Build history of the part. All positions in model axes, mm. A direction names the side the tool comes from. Coordinates: 2 decimals unless noted, no trailing zeros. Order: outer loops, then holes, each group sorted by start corner. A loop starts at its lowest first (then second) coordinate and runs counter-clockwise, first axis right, second up. Notation, with made-up numbers: M -29.75,-24.5 L -6.75,-24.5 A19 cw -6.75,-19.5 Z; hole C 18.5,32 d11. An arc over 180 degrees is marked long. Use a Markdown table: item, result. Add a question column.
from build123d import *

# Parameters (mm, degrees)
BOSS_EXTRUDE1_DEPTH = 152.4
BOSS_EXTRUDE2_DEPTH = 12.7
SKETCH3_R           = 2.5
CUT_EXTRUDE1_DEPTH  = 25
SKETCH4_R           = 3.5
CUT_EXTRUDE2_DEPTH  = 2


with BuildPart() as part:
    # Sketch1 → Boss-Extrude1 (new body)
    with BuildSketch(Plane(origin=(0, 0, 0), x_dir=(0, 1, 0), z_dir=(0, 0, 1))):
        with BuildLine():
            Line((-94.231538291, 5), (-88.9, 5))
            Line((-88.9, 5), (-88.9, 19.05))
            Line((-88.9, 19.05), (-215.9, 19.05))
            Line((-215.9, 19.05), (-215.9, -7.7))
            ThreePointArc((-215.9, -7.7), (-208.57766953, -25.37766953), (-190.9, -32.7))
            Line((-190.9, -32.7), (-152.8, -32.7))
            Line((-152.8, -32.7), (-152.8, -20))
            Line((-152.8, -20), (-170.3, -20))
            ThreePointArc((-170.3, -20), (-175.603300859, -17.803300859), (-177.8, -12.5))
            Line((-177.8, -12.5), (-177.8, -7.5))
            ThreePointArc((-177.8, -7.5), (-175.603300859, -2.196699141), (-170.3, 0))
            Line((-170.3, 0), (-141.9, 0))
            Line((-141.9, 0), (-144.231538291, 5))
            Line((-144.231538291, 5), (-133.568461709, 5))
            Line((-133.568461709, 5), (-135.9, 0))
            Line((-135.9, 0), (-91.9, 0))
            Line((-91.9, 0), (-94.231538291, 5))
        make_face()
        with BuildLine():
            Line((-35.9, 0), (-7.5, 0))
            ThreePointArc((-7.5, 0), (-2.196699141, -2.196699141), (0, -7.5))
            Line((0, -7.5), (0, -12.5))
            ThreePointArc((0, -12.5), (-2.196699141, -17.803300859), (-7.5, -20))
            Line((-7.5, -20), (-25, -20))
            Line((-25, -20), (-25, -32.7))
            Line((-25, -32.7), (13.1, -32.7))
            ThreePointArc((13.1, -32.7), (30.77766953, -25.37766953), (38.1, -7.7))
            Line((38.1, -7.7), (38.1, 19.05))
            Line((38.1, 19.05), (-88.9, 19.05))
            Line((-88.9, 19.05), (-88.9, 5))
            Line((-88.9, 5), (-83.568461709, 5))
            Line((-83.568461709, 5), (-85.9, 0))
            Line((-85.9, 0), (-41.9, 0))
            Line((-41.9, 0), (-44.231538291, 5))
            Line((-44.231538291, 5), (-33.568461709, 5))
            Line((-33.568461709, 5), (-35.9, 0))
        make_face()
    extrude(amount=BOSS_EXTRUDE1_DEPTH)

    # Sketch2 → Boss-Extrude2 (add)
    with BuildSketch(Plane(origin=(0, 0, 0), x_dir=(1, 0, 0), z_dir=(0, 0, -1))):
        Polygon((-19.05, 215.9), (-19.05, -38.1), (7.7, -38.1), (32.7, 25), (32.7, 152.8), (32.7, 190.9), (7.7, 215.9), align=None)
    extrude(amount=-BOSS_EXTRUDE2_DEPTH)

    # Sketch3 → Cut-Extrude1 (cut)
    with BuildSketch(Plane.YZ):
        with Locations(Location((-107.285735893, 82.55, 0), (0, 0, 270))):
            Circle(SKETCH3_R)
        with Locations(Location((-107.285735893, 127.55, 0), (0, 0, 270))):
            Circle(SKETCH3_R)
        with Locations(Location((-107.285735893, 37.55, 0), (0, 0, 270))):
            Circle(SKETCH3_R)
        with Locations(Location((-70.514264107, 37.55, 0), (0, 0, 180))):
            Circle(SKETCH3_R)
        with Locations(Location((-70.514264107, 82.55, 0), (0, 0, 180))):
            Circle(SKETCH3_R)
        with Locations(Location((-70.514264107, 127.55, 0), (0, 0, 180))):
            Circle(SKETCH3_R)
    extrude(amount=-CUT_EXTRUDE1_DEPTH, mode=Mode.SUBTRACT)

    # Sketch4 → Cut-Extrude2 (cut)
    with BuildSketch(Plane.YZ):
        with Locations(Location((-107.285735893, 127.55, 0), (0, 0, 270))):
            Circle(SKETCH4_R)
        with Locations(Location((-107.285735893, 82.55, 0), (0, 0, 270))):
            Circle(SKETCH4_R)
        with Locations(Location((-107.285735893, 37.55, 0), (0, 0, 270))):
            Circle(SKETCH4_R)
        with Locations(Location((-70.514264107, 37.55, 0), (0, 0, 270))):
            Circle(SKETCH4_R)
        with Locations(Location((-70.514264107, 82.55, 0), (0, 0, 270))):
            Circle(SKETCH4_R)
        with Locations(Location((-70.514264107, 127.55, 0), (0, 0, 270))):
            Circle(SKETCH4_R)
    extrude(amount=-CUT_EXTRUDE2_DEPTH, mode=Mode.SUBTRACT)


solid = part.part
(1) Slice it at C-C on z = 37.55. State how many separate pieces and enclosed holes the cut face has, and give its area (3 significant figures).
(2) Slice it at D-D on x = 22.5. Give the cut face in (y, z), and give its area (3 significant figures).
(3) Mould opens along Z. For faces 1 (the flat face through (-11, -91, 152.4)), 2 (the flat face through (26, -152.8, 82)), 3 (the flat face through (-2, -106, 85)) say: released by +Z, released by -Z, zero draft, split by the parting line, or undercut.
(4) Drop flat-ended pins along their axis: P1, Ø8.5, axis at y = -41, z = 107.5, coming from the +X side; P2, Ø1.5, axis at x = 14.5, z = 39, coming from the +Y side; P3, Ø12, axis at x = 23, z = 98, coming from the -Y side. Give the stop position or say it passes through.
(5) Which spindle directions (+Z, -Z, +X, -X, +Y, -Y) get a long thin tool onto all of the face, cutting with end or side? Do faces 4 (the flat face through (10, -177.8, 82)), 5 (the flat face through (0, -64, 82)), 6 (the cylindrical face through (-0.99, -67.56, 35.67)), 7 (the cylindrical face through (-10.41, -68.67, 35.86)). Say none if no direction does.
(6) Drill centre lines: line 1 along X through (y, z) = (-18.5, 75); line 2 along Y through (x, z) = (-4, 135); line 3 along Y through (x, z) = (-4.5, 138.5). Where is each one in solid material? Low to high. Write a range as from..to.
(7) Slice it at B-B on y = -19.5. Give the cut face in (x, z), and give its area (3 significant figures).
Solutions:
| question | item | result |
|---|---|---|
| 1 | separate pieces | 3 |
| 1 | enclosed holes | 0 |
| 1 | area | 7,420 mm² |
| 2 | outline | M -211.05,0 L 33.25,0 L 33.25,152.4 L -25,152.4 L -25,12.7 L -152.8,12.7 L -152.8,152.4 L -211.05,152.4 Z |
| 2 | area | 19,400 mm² |
| 3 | face 1 | released by +Z |
| 3 | face 2 | zero draft |
| 3 | face 3 | undercut |
| 4 | P1 | x = 0 |
| 4 | P2 | y = 37.36 |
| 4 | P3 | y = -214.11 |
| 5 | face 4 | +Z |
| 5 | face 5 | +Z, +X |
| 5 | face 6 | +X |
| 5 | face 7 | +X, -X |
| 6 | line 1 | -19.05..0, 20..32.7 |
| 6 | line 2 | -215.9..-143.77, -134.03..-93.77, -84.03..-43.77, -34.03..38.1 |
| 6 | line 3 | -215.9..-144, -133.8..-94, -83.8..-44, -33.8..38.1 |
| 7 | outline | M -19.05,0 L 32.7,0 L 32.7,152.4 L 20,152.4 L 20,12.7 L 0,12.7 L 0,152.4 L -19.05,152.4 Z |
| 7 | area | 5,090 mm² |
